Autodesk Fusion 360 part; units mm, degrees
sketch "Sketch1" plane through (0, 0, 0) normal (0, 0, 1) x (1, 0, 0)
  line L0 (50, -50) -> (-50, -50)
  line L1 (-50, -50) -> (-50, 50)
  line L2 (-50, 50) -> (50, 50)
  line L3 (50, 50) -> (50, -50)
  line L4 (50, -50) -> (-50, 50) construction
  line L5 (-50, -50) -> (50, 50) construction
  dimension "d1" = 100
  dimension "d2" = 100
extrude "Extrude1" add sketch "Sketch1" along normal blind 20
sketch "Sketch2" plane through (0, 0, 20) normal (0, 0, 1) x (-1, 0, 0)
  line L0 (-50, -50) -> (50, -50)
  line L1 (50, -50) -> (50, 50)
  line L2 (50, 50) -> (-50, 50)
  line L3 (-50, 50) -> (-50, -50)
  circle A0 centre (0, 0) radius 50
extrude "Extrude2" add sketch "Sketch2" along normal blind 5 contours A0
sketch "Sketch3" plane through (0, 0, 25) normal (0, 0, 1) x (-1, 0, 0)
  circle A0 centre (0, 0) radius 50
  circle A1 centre (0, 0) radius 35
  dimension "d7" = 70
extrude "Extrude3" add sketch "Sketch3" along normal blind 5 contours A1
sketch "Sketch4" plane through (0, 0, 30) normal (0, 0, 1) x (-1, 0, 0)
  circle A0 centre (0, 0) radius 35
  circle A1 centre (0, 0) radius 25 construction
  arc A2 (0, -30) -> (0, -20) centre (0, -25) ccw
  arc A3 (-10.8928, -16.7734) -> (-16.3392, -25.1601) centre (-13.616, -20.9668) ccw
  arc A4 (-10.8928, -16.7734) -> (0, -20) centre (0, 0) ccw
  arc A5 (-16.3392, -25.1601) -> (0, -30) centre (0, 0) ccw
  arc A6 (25.9808, 15) -> (17.3205, 10) centre (21.6506, 12.5) ccw
  arc A7 (19.9726, -1.0467) -> (29.9589, -1.5701) centre (24.9657, -1.3084) ccw
  arc A8 (19.9726, -1.0467) -> (17.3205, 10) centre (0, 0) ccw
  arc A9 (29.9589, -1.5701) -> (25.9808, 15) centre (0, 0) ccw
  arc A10 (-25.9808, 15) -> (-17.3205, 10) centre (-21.6506, 12.5) ccw
  arc A11 (-9.0798, 17.8201) -> (-13.6197, 26.7302) centre (-11.3498, 22.2752) ccw
  arc A12 (-9.0798, 17.8201) -> (-17.3205, 10) centre (0, 0) ccw
  arc A13 (-13.6197, 26.7302) -> (-25.9808, 15) centre (0, 0) ccw
  dimension "d11" = 40
  dimension "d12" = 60
  dimension "d13" = 50
  dimension "d16" = 360
extrude "Extrude4" cut sketch "Sketch4" against normal blind 5 contours A2 A3 A4 A5 | A6 A7 A8 A9 | A10 A11 A12 A13
sketch "Sketch5" plane through (0, 0, 30) normal (0, 0, 1) x (-1, 0, 0)
  arc A0 (-13.6197, 26.7302) -> (-25.9808, 15) centre (0, 0) ccw
  arc A1 (-9.0798, 17.8201) -> (-13.6197, 26.7302) centre (-11.3498, 22.2752) ccw
  arc A2 (-9.0798, 17.8201) -> (-17.3205, 10) centre (0, 0) ccw
  arc A3 (-25.9808, 15) -> (-17.3205, 10) centre (-21.6506, 12.5) ccw
  arc A4 (-16.3392, -25.1601) -> (0, -30) centre (0, 0) ccw
  arc A5 (-10.8928, -16.7734) -> (-16.3392, -25.1601) centre (-13.616, -20.9668) ccw
  arc A6 (-10.8928, -16.7734) -> (0, -20) centre (0, 0) ccw
  arc A7 (0, -30) -> (0, -20) centre (0, -25) ccw
  arc A8 (29.9589, -1.5701) -> (25.9808, 15) centre (0, 0) ccw
  arc A9 (19.9726, -1.0467) -> (29.9589, -1.5701) centre (24.9657, -1.3084) ccw
  arc A10 (19.9726, -1.0467) -> (17.3205, 10) centre (0, 0) ccw
  arc A11 (25.9808, 15) -> (17.3205, 10) centre (21.6506, 12.5) ccw
  circle A12 centre (0, 0) radius 35
sketch "Sketch6" plane through (0, 0, 30) normal (0, 0, 1) x (1, 0, 0)
  circle A0 centre (0, 0) radius 15
  dimension "d19" = 30
extrude "Extrude5" cut sketch "Sketch6" against normal blind 10
sketch "Sketch7" plane through (0, 0, 25) normal (0, 0, 1) x (-1, 0, 0)
  circle A0 centre (0, 0) radius 35
  circle A1 centre (0, 0) radius 50
  circle A2 centre (0, 0) radius 41.5 construction
  line L0 (0, 0) -> (50, 0) construction
  circle A3 centre (41.5, 0) radius 4
  circle A4 centre (0, 41.5) radius 4
  circle A5 centre (-41.5, 0) radius 4
  circle A6 centre (0, -41.5) radius 4
  dimension "d22" = 83
  dimension "d23" = 8
  dimension "d25" = 360
extrude "Extrude6" cut sketch "Sketch7" against normal blind 5 contours A3 | A4 | A5 | A6
CAD build for the part. Positions are in the model's coordinates, mm. A direction names the side the tool comes from. Coordinates: 2 decimals unless noted, no trailing zeros. Write each loop counter-clockwise with the first axis right and the second up, starting at its lowest first coordinate (ties: lowest second). Pieces come first, ordered by that corner, then holes. Notation, with made-up numbers: (41, 27) - (57, 27) arc R21 ccw to (57, 38) - close; hole circle Ø11 at (35.25, -22). An arc over 180 degrees is marked (long way). Use a Markdown table: item, result. Add a question column.
Item 1: Drill centre lines: L1, parallel to Y at x = 0, z = 21.25; L2, parallel to X at y = 5, z = 25.75; L3, parallel to Y at x = 7, z = 26.75 (1 decimal). Where is each one in solid material? Low to high. Write a range as from..to.
Item 2: 3-axis set-ups, long thin cutter, end or side, ignore diameter. For faces 1 (the face through (42, 0, 20)), 2 (the face through (-40, -38, 20)), 3 (the face through (50, 1, 10)), 4 (the face through (40, -40, 20)): which of +Z, -Z, +X, -X, +Y, -Y reach the whole face in a straight line?
Item 3: Mould opens along Y. For faces 5 (the face through (24.2, -8.2, 27.5)), 6 (the face through (-47.69, 15.02, 22.46)), 7 (the face through (0, 41, 20)), 8 (the face through (-1, 50, 10)) say: pulls with the +Y half, pulls with the -Y half, needs draft (parallel to the pull), parting line crosses it, or undercut.
Item 4: Band-saw the part on B-B, the plane x = 41.5. Give the cut face in (y, z), and give its area (3 significant figures).
Item 5: Flat gauge pins, fed straight in: pin 1 (25 mm diameter, centred on x = -37, y = -33, fed in from +Z); pin 2 (2.5 mm diameter, centred on x = -41, y = -1, fed in from +Z); pin 3 (1 mm diameter, centred on y = -36, z = 23.5, fed in from +X). Where does each tip first touch, or does it go through?
Item 6: Band-saw the part on C-C, the plane y = 18.5. Give the cut face in (x, z).
Item 7: Band-saw the part on A-A, the plane y = -30. Give the cut face in (x, z).
Numbers:
| question | item | result |
|---|---|---|
| 1 | L1 | -50..-45.5, -37.5..-15, 15..37.5, 45.5..50 |
| 1 | L2 | -34.64..-28.34, -21.59..-14.14, 14.14..34.64 |
| 1 | L3 | -34.3..-24.7, -19.8..-13.3, 13.3..18.7, 29.2..34.3 |
| 2 | face 1 | +Z |
| 2 | face 2 | +Z, -X, -Y |
| 2 | face 3 | +Z, -Z, +X, +Y, -Y |
| 2 | face 4 | +Z, +X, -Y |
| 3 | face 5 | undercut |
| 3 | face 6 | parting line crosses it |
| 3 | face 7 | undercut |
| 3 | face 8 | pulls with the +Y half |
| 4 | outline | (-50, 0) - (50, 0) - (50, 20) - (27.89, 20) - (27.89, 25) - (4, 25) - (4, 20) - (-4, 20) - (-4, 25) - (-27.89, 25) - (-27.89, 20) - (-50, 20) - close |
| 4 | area | 2,240 mm2 |
| 5 | pin 1 | z = 25 |
| 5 | pin 2 | z = 20 |
| 5 | pin 3 | x = 35.21 |
| 6 | outline | (-50, 0) - (50, 0) - (50, 20) - (46.45, 20) - (46.45, 25) - (29.71, 25) - (29.71, 30) - (17.97, 30) - (17.97, 25) - (7.6, 25) - (7.6, 30) - (-29.71, 30) - (-29.71, 25) - (-46.45, 25) - (-46.45, 20) - (-50, 20) - close |
| 7 | outline | (-50, 0) - (50, 0) - (50, 20) - (40, 20) - (40, 25) - (18.03, 25) - (18.03, 30) - (-18.03, 30) - (-18.03, 25) - (-40, 25) - (-40, 20) - (-50, 20) - close |
